The drawing under review shows one solid part. Ordinate dimensions are in mm from its lowest x, y, z. Coordinates: 2 decimals unless noted, no trailing zeros. Order: outer loops, then holes, each group sorted by start corner. A loop starts at its lowest first (then second) coordinate and runs counter-clockwise, first axis right, second up. Notation, with made-up numbers: M 84.25,-25.5 L 100.25,-25.5 A20 ccw 100.25,1.5 Z; hole C -29.75,31.25 d2. An arc over 180 degrees is marked long. Answer as a JSON object with one key per item and string values.
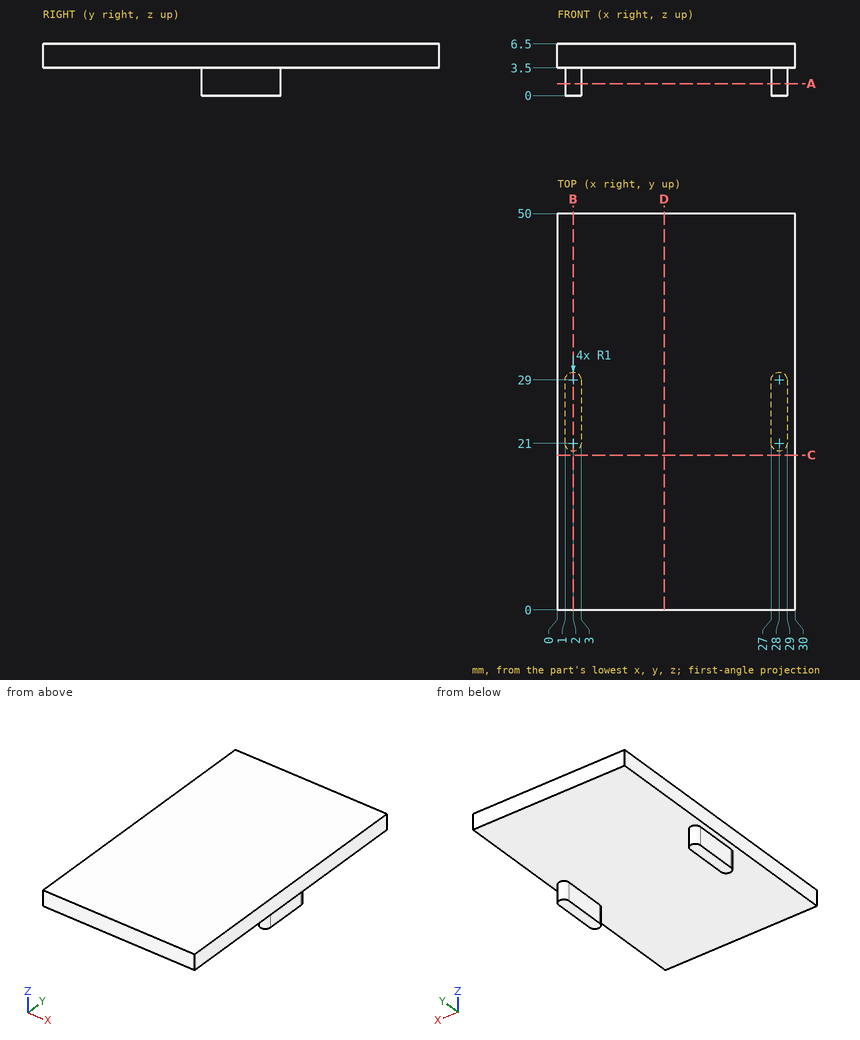
1) Add section D-D (x = 13.5). State the section outline as (y, z) points.
Taken from the geometry:
{"outline": "M 0,3.5 L 50,3.5 L 50,6.5 L 0,6.5 Z"}
2) Add section A-A (z = 1.5). State the section outline as (x, y) points, and give its area (3 significant figures).
Taken from the geometry:
{"outline": "M 1,21 A1 ccw 3,21 L 3,29 A1 ccw 1,29 Z; M 27,21 A1 ccw 29,21 L 29,29 A1 ccw 27,29 Z", "area": "38.3 mm2"}
3) Add section B-B (x = 2). State the section outline as (y, z) points.
Taken from the geometry:
{"outline": "M 0,3.5 L 20,3.5 L 20,0 L 30,0 L 30,3.5 L 50,3.5 L 50,6.5 L 0,6.5 Z"}
4) Insertion check: pin 1 Ø10 at (x, y) = (10.5, 7.5) entering from -Z; pin 2 Ø3 at (y, z) = (26.5, 1.5) entering from -X. Each pin has a flat end and moves straight along its axis. Give the tip position at first contact, or say it passes through.
Taken from the geometry:
{"pin 1": "stops at z = 3.5", "pin 2": "stops at x = 1"}
5) Add section C-C (y = 19.5). State the section outline as (x, z) points.
Taken from the geometry:
{"outline": "M 0,3.5 L 30,3.5 L 30,6.5 L 0,6.5 Z"}
6) To check wall thickness, follow L1, parallel to X at y = 24.5, z = 1; L2, parallel to Z at x = 19.25, y = 30; L3, parallel to Y at x = 28, z = 1.5. State the ranges of each line that lie inside material, in increasing order.
Taken from the geometry:
{"L1": "x = 1 to 3, 27 to 29", "L2": "z = 3.5 to 6.5", "L3": "y = 20 to 30"}
